Part model, mm, in its own coordinate system. A direction names the side the tool comes from. Coordinates: 2 decimals unless noted, no trailing zeros. Write each loop counter-clockwise with the first axis right and the second up, starting at its lowest first coordinate (ties: lowest second). Pieces come first, ordered by that corner, then holes. Notation, with made-up numbers: (11.5, 49) - (19.5, 49) arc R22 ccw to (19.5, 74) - close; hole circle Ø9 at (64, -34.5). An arc over 180 degrees is marked (long way). Use a Markdown table: item, result.
```python
from build123d import *

# Parameters (mm, degrees)
BOSS_EXTRUDE1_DEPTH      = 10
CUT_EXTRUDE3_DEPTH       = 17
SKETCH5_R                = 2.2
CUT_EXTRUDE4_DEPTH       = 11
FILLET2_R                = 4
SKETCH7_R                = 5
SKETCH7_R_2              = 2.2
BOSS_EXTRUDE2_DEPTH      = 0.5
BOSS_EXTRUDE2_DEPTH_BACK = 3
SKETCH8_W                = 15.12
SKETCH8_H                = 0.88
BOSS_EXTRUDE3_DEPTH      = 0.8
SKETCH9_W                = 15.12
SKETCH9_H                = 1.76
BOSS_EXTRUDE4_DEPTH      = 3.3


with BuildPart() as part:
    # Sketch1 → Boss-Extrude1 (new body)
    with BuildSketch(Plane.XY):
        with BuildLine():
            Line((-5, 7.5), (-5, -4.5))
            ThreePointArc((-5, -4.5), (3, -12.5), (11, -4.5))
            Line((11, -4.5), (11, 7.5))
            ThreePointArc((11, 7.5), (3, 15.5), (-5, 7.5))
        make_face()
    extrude(amount=BOSS_EXTRUDE1_DEPTH)

    # Sketch4 → Cut-Extrude3 (cut, through all)
    with BuildSketch(Plane.ZY.offset(5)):
        with BuildLine():
            Line((6.641476618, -0.851663389), (5.9, 0.207274966))
            Line((5.9, 0.207274966), (5.9, 2.792725034))
            Line((5.9, 2.792725034), (6.641476618, 3.851663389))
            ThreePointArc((6.641476618, 3.851663389), (14.1, 1.5), (6.641476618, -0.851663389))
        make_face()
    extrude(amount=-CUT_EXTRUDE3_DEPTH, mode=Mode.SUBTRACT)

    # Sketch5 → Cut-Extrude4 (cut, through all)
    with BuildSketch(Plane(origin=(0, 0, 0), x_dir=(-1, 0, 0), z_dir=(0, 0, -1))):
        with Locations((-3, 8.5)):
            Circle(SKETCH5_R)
        with Locations((-3, -5.5)):
            Circle(SKETCH5_R)
    extrude(amount=-CUT_EXTRUDE4_DEPTH, mode=Mode.SUBTRACT)

    # Fillet2
    fillet2_edges = [part.edges().sort_by_distance(p)[0] for p in [
        (-5, 1.5, 0),
        (3, 15.5, 0),
        (11, 1.5, 0),
        (3, -12.5, 0),
    ]]
    fillet(fillet2_edges, radius=FILLET2_R)

    # Sketch7 → Boss-Extrude2 (add, two sides)
    with BuildSketch(Plane(origin=(0, 0, 0), x_dir=(-1, 0, 0), z_dir=(0, 0, -1))) as boss_extrude2_sk:
        with Locations((-3, 8.5)):
            Circle(SKETCH7_R)
        with Locations((-3, 8.5)):
            Circle(SKETCH7_R_2, mode=Mode.SUBTRACT)
        with Locations((-3, -5.5)):
            Circle(SKETCH7_R)
        with Locations((-3, -5.5)):
            Circle(SKETCH7_R_2, mode=Mode.SUBTRACT)
    extrude(amount=BOSS_EXTRUDE2_DEPTH)
    extrude(boss_extrude2_sk.sketch, amount=-BOSS_EXTRUDE2_DEPTH_BACK)

    # Sketch8 → Boss-Extrude3 (add)
    with BuildSketch(Plane.XY.offset(5.9)):
        with Locations((3, 1.5)):
            Rectangle(SKETCH8_W, SKETCH8_H)
    extrude(amount=BOSS_EXTRUDE3_DEPTH)

    # Sketch9 → Boss-Extrude4 (add)
    with BuildSketch(Plane.XY.offset(6.7)):
        with Locations((3, 1.5)):
            Rectangle(SKETCH9_W, SKETCH9_H)
    extrude(amount=BOSS_EXTRUDE4_DEPTH)


solid = part.part
```
Item 1: Two-plate mould, pull along Y, no slides. Class faces 1 (the face through (2.824, -12.498, 6.958)), 2 (the face through (3, -9, 10)), 3 (the face through (2.888, 5.124, 8.082)): pulls with the +Y half, pulls with the -Y half, needs draft (parallel to the pull), parting line crosses it, or undercut.
From the geometry:
| item | result |
|---|---|
| face 1 | pulls with the -Y half |
| face 2 | needs draft |
| face 3 | undercut |
Item 2: Drill centre lines: probe 1 along Y at (x, z) = (3, 5.5); probe 2 along Y at (x, z) = (3, -0.15); probe 3 along Y at (x, z) = (4, 3). Where is each one in solid material? Low to high.
From the geometry:
| item | result |
|---|---|
| probe 1 | -12.5 to -7.7, -3.3 to 6.3, 10.7 to 15.5 |
| probe 2 | -10.5 to -7.7, -3.3 to -0.5, 3.5 to 6.3, 10.7 to 13.5 |
| probe 3 | -12.31 to -7.46, -3.54 to 6.54, 10.46 to 15.31 |
Item 3: Band-saw the part on A-A, the plane z = 7. Give the cut face in (x, y), then the cut area to 3 significant figures.
From the geometry:
| item | result |
|---|---|
| outline | (-5, -4.5) arc R8 ccw to (11, -4.5) - (11, -1.29) - (-5, -1.29) - close; (-5, 4.29) - (11, 4.29) - (11, 7.5) arc R8 ccw to (-5, 7.5) - close; (-4.56, 0.62) - (10.56, 0.62) - (10.56, 2.38) - (-4.56, 2.38) - close; hole circle Ø4.4 at (3, -5.5); hole circle Ø4.4 at (3, 8.5) |
| area | 300 mm^2 |
Item 4: Drop flat-ended pins along their axis: P1, Ø3.5, axis at x = 3, y = 8.5, coming from the -Z side; P2, Ø4, axis at x = 0, z = 2.5, coming from the +Y side; P3, Ø1.4, axis at y = 1.5, z = 8, coming from the +X side; P4, Ø3.5, axis at x = 5.5, z = 9, coming from the -Y side. Give the stop position or say it passes through.
From the geometry:
| item | result |
|---|---|
| P1 | through |
| P2 | y = 15.37 |
| P3 | x = 10.56 |
| P4 | y = -12.46 |
Item 5: Band-saw the part on C-C, the plane z = 5. Give the cut face in (x, y), then the cut area to 3 significant figures.
From the geometry:
| item | result |
|---|---|
| outline | (-5, -4.5) arc R8 ccw to (11, -4.5) - (11, 7.5) arc R8 ccw to (-5, 7.5) - close; hole circle Ø4.4 at (3, -5.5); hole circle Ø4.4 at (3, 8.5) |
| area | 363 mm^2 |
Item 6: Which spindle directions (+Z, -Z, +X, -X, +Y, -Y) get a long thin tool onto all of the face, cutting with end or side? Do faces 4 (the face through (-4.56, 1, 8)), 5 (the face through (-5, 1.6, 5.6)), 6 (the face through (2.888, 3.315, 6.266)). Say none if no direction does.
From the geometry:
| item | result |
|---|---|
| face 4 | +Z, -X |
| face 5 | +Z, -Z, -X, +Y, -Y |
| face 6 | +Z, +X, -X |
Item 7: Band-saw the part on B-B, the plane x = 3. Count the separate pieces of the cut face and the enclosed holes in it, then the cut area to 3 significant figures.
From the geometry:
| item | result |
|---|---|
| separate pieces | 3 |
| enclosed holes | 0 |
| area | 171 mm^2 |
